Geometry check sheet. Reference: the model listing, model coordinates, mm. Face numbers are marked on the shaded views. A direction names the side the tool comes from. Coordinates: 2 decimals unless noted, no trailing zeros. Order: outer loops, then holes, each group sorted by start corner. A loop starts at its lowest first (then second) coordinate and runs counter-clockwise, first axis right, second up. Notation, with made-up numbers: (6, -20.75) - (43, -20.75) arc R21 ccw to (43, 7.25) - close; hole circle Ø1 at (40, 37). An arc over 180 degrees is marked (long way). Put each result on its own line as item: value.
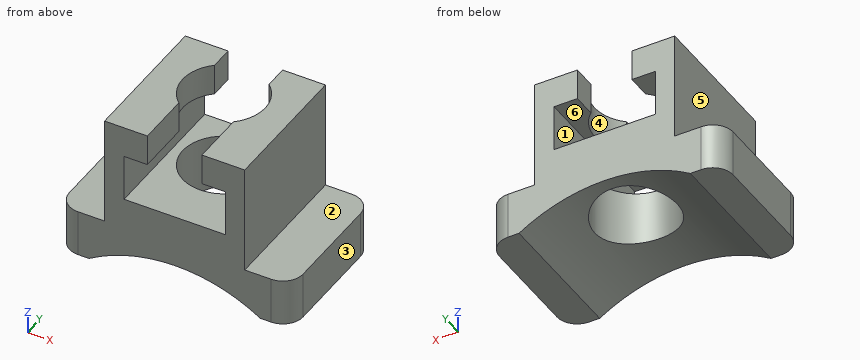
from build123d import *

# Parameters (mm, degrees)
PAD_DEPTH         = 30
SKETCH002_W       = 90
SKETCH002_H       = 90
PAD001_DEPTH      = 100
POCKET_DEPTH      = 45.001
POCKET_DEPTH_BACK = -45.001
POCKET001_DEPTH   = 90.001
SKETCH004_R       = 26.5
POCKET002_DEPTH   = 100.001


with BuildPart() as part:
    # Sketch (on XY_Plane of Origin) → Pad (new body)
    with BuildSketch(Plane.XY):
        with BuildLine():
            Line((-75, 32), (-75, -32))
            ThreePointArc((-75, -32), (-71.192388, -41.192388), (-62, -45))
            Line((-62, -45), (62, -45))
            ThreePointArc((62, -45), (71.192388, -41.192388), (75, -32))
            Line((75, -32), (75, 32))
            ThreePointArc((75, 32), (71.192388, 41.192388), (62, 45))
            Line((62, 45), (-62, 45))
            ThreePointArc((-62, 45), (-71.192388, 41.192388), (-75, 32))
        make_face()
    extrude(amount=PAD_DEPTH)

    # Sketch002 (on XY_Plane of Origin) → Pad001 (join)
    with BuildSketch(Plane.XY):
        Rectangle(SKETCH002_W, SKETCH002_H)
    extrude(amount=PAD001_DEPTH)

    # Sketch001 (on XZ_Plane of Origin) → Pocket (cut, two sides)
    with BuildSketch(Plane.XZ) as pocket_sk:
        with BuildLine():
            ThreePointArc((55, 0), (0, 16), (-55, 0))
            Line((-55, 0), (55, 0))
        make_face()
    extrude(amount=-POCKET_DEPTH, mode=Mode.SUBTRACT)
    extrude(pocket_sk.sketch, amount=-POCKET_DEPTH_BACK, mode=Mode.SUBTRACT)

    # Sketch003 (on Face14 of Pocket) → Pocket001 (cut, through all)
    with BuildSketch(Plane.XZ.offset(45)):
        Polygon((-17.5, 100), (17.5, 100), (17.5, 80), (32.5, 80), (32.5, 50), (-32.5, 50), (-32.5, 80), (-17.5, 80), align=None)
    extrude(amount=-POCKET001_DEPTH, mode=Mode.SUBTRACT)

    # Sketch004 (on XY_Plane of Origin) → Pocket002 (cut, through all)
    with BuildSketch(Plane.XY):
        with Locations((0, 10)):
            Circle(SKETCH004_R)
    extrude(amount=POCKET002_DEPTH, mode=Mode.SUBTRACT)


solid = part.part
Q1. Depth check by flat-ended pin: pin 1 Ø24 at (y, z) = (22.5, 64.5) entering from +X; pin 2 Ø12 at (x, y) = (27.5, 23) entering from -Z; pin 3 Ø12 at (x, y) = (19, -20.5) entering from -Z. Enter the tip coordinate at first touch or a pass-through.
Answer block:
pin 1: stops at x = 45
pin 2: stops at z = 10.37
pin 3: stops at z = 12.91
Q2. Draft check along Z on the marked faces 1, 2 and 3. Enter one of: pulls with the +Z half, pulls with the -Z half, needs draft (parallel to the pull), parting line crosses it, or undercut.
Answer block:
face 1: undercut
face 2: pulls with the +Z half
face 3: needs draft
Q3. Access from +Z, -Z, +X, -X, +Y, -Y to the whole of each face (thin tool, end or side, straight path). Record for the marked faces 4, 5 and 6.
Answer block:
face 4: +Z, -Z
face 5: +Z, -X, +Y, -Y
face 6: +Y, -Y
Q4. Section check D-D on y = -19.5. Record the boundary of the cut face in (x, z).
Answer block:
outline: (-75, 0) - (-55, 0) arc R102.53 cw to (55, 0) - (75, 0) - (75, 30) - (45, 30) - (45, 100) - (17.5, 100) - (17.5, 80) - (32.5, 80) - (32.5, 50) - (-32.5, 50) - (-32.5, 80) - (-17.5, 80) - (-17.5, 100) - (-45, 100) - (-45, 30) - (-75, 30) - close
Q5. Section check C-C on y = 10. Record the boundary of the cut face in (x, z).
Answer block:
outline: (-75, 0) - (-55, 0) arc R102.53 cw to (-26.5, 12.52) - (-26.5, 50) - (-32.5, 50) - (-32.5, 80) - (-26.5, 80) - (-26.5, 100) - (-45, 100) - (-45, 30) - (-75, 30) - close; (26.5, 12.52) arc R102.53 cw to (55, 0) - (75, 0) - (75, 30) - (45, 30) - (45, 100) - (26.5, 100) - (26.5, 80) - (32.5, 80) - (32.5, 50) - (26.5, 50) - close
Q6. Thickness scan on L1, parallel to Y at x = 0, z = 20.5; L2, parallel to X at y = -25, z = 76; L3, parallel to X at y = 10, z = 23. Record the ranges inside material, lowest first. Write a range as [from, to].
Answer block:
L1: y = [-45, -16.5], [36.5, 45]
L2: x = [-45, -32.5], [32.5, 45]
L3: x = [-75, -26.5], [26.5, 75]
Q7. Section check B-B on x = 0. Record the boundary of the cut face in (y, z), then the cut area to 3 significant figures.
Answer block:
outline: (-45, 16) - (-16.5, 16) - (-16.5, 50) - (-45, 50) - close; (36.5, 16) - (45, 16) - (45, 50) - (36.5, 50) - close
area: 1,260 mm^2
Q8. Section check A-A on z = 69. Record the boundary of the cut face in (x, y).
Answer block:
outline: (-45, -45) - (-32.5, -45) - (-32.5, 45) - (-45, 45) - close; (32.5, -45) - (45, -45) - (45, 45) - (32.5, 45) - close
